Verification items for the finished model (mm, model axes). A direction names the side the tool comes from. Coordinates: 2 decimals unless noted, no trailing zeros. Order: outer loops, then holes, each group sorted by start corner. A loop starts at its lowest first (then second) coordinate and runs counter-clockwise, first axis right, second up. Notation, with made-up numbers: (63.25, 78.25) -> (104.25, 78.25) arc R29 cw to (104.25, 100.25) -> close; hole circle Ø3 at (-6, 8.25). An arc over 180 degrees is marked (long way). Answer as CSV lines item,"result".
```python
from build123d import *

# Parameters (mm, degrees)
F0_W      = 100
F0_H      = 100
F1_DEPTH  = 2
F2_R      = 7.5
F2_W      = 50.5
F2_H      = 2.1
F3_DEPTH  = 25
F4_W      = 8.5
F4_H      = 100
F4_W_2    = 3.5
F4_H_2    = 49
F5_DEPTH  = 25
F6_W      = 8.5
F6_H      = 8.5
F7_DEPTH  = 56.75
F8_W      = 2.5
F8_H      = 50
F9_DEPTH  = 5.2
F10_R     = 1
F11_W     = 1
F11_H     = 2.1
F11_W_2   = 3.33
F12_DEPTH = 4.5


# Not quite as in the source:
# - a pattern or mirror of a feature is missing from the dataset's text; its kind, count and spacing are read off the source's solid


with BuildPart() as f1:
    # F0 (on Top) → F1 (new body)
    with BuildSketch(Plane.XY):
        Rectangle(F0_W, F0_H)
    extrude(amount=F1_DEPTH)

    # F2 (on face) → F3 (cut)
    with BuildSketch(Plane.XY.offset(2)):
        with BuildLine():
            ThreePointArc((-21.1883002739, 41.0541145875), (-23.9038135596, 39.3292567737), (-23.4967439726, 36.1381063176))
            Line((-23.4967439726, 36.1381063176), (-8.2072148474, 17.7169868897))
            ThreePointArc((-8.2072148474, 17.7169868897), (-6.7654738079, 16.7609181236), (-5.0355363465, 16.7598739167))
            ThreePointArc((-5.0355363465, 16.7598739167), (0, 17.5), (5.0355363465, 16.7598739167))
            ThreePointArc((5.0355363465, 16.7598739167), (6.7654738079, 16.7609181236), (8.2072148474, 17.7169868897))
            Line((8.2072148474, 17.7169868897), (23.4967439726, 36.1381063176))
            ThreePointArc((23.4967439726, 36.1381063176), (23.9038135596, 39.3292567737), (21.1883002739, 41.0541145875))
            Line((21.1883002739, 41.0541145875), (-21.1883002739, 41.0541145875))
        make_face()
        with BuildLine():
            ThreePointArc((-15.5455239175, -8.0365842327), (-17.5, 0), (-15.5455239175, 8.0365842327))
            ThreePointArc((-15.5455239175, 8.0365842327), (-15.2278910436, 9.7371118179), (-15.9020271762, 11.3302926568))
            Line((-15.9020271762, 11.3302926568), (-31.1915563014, 29.7514120847))
            ThreePointArc((-31.1915563014, 29.7514120847), (-34.5184961718, 30.6572233604), (-36.5, 27.8354038148))
            Line((-36.5, 27.8354038148), (-36.5, -27.8354038148))
            ThreePointArc((-36.5, -27.8354038148), (-34.5184961718, -30.6572233604), (-31.1915563014, -29.7514120847))
            Line((-31.1915563014, -29.7514120847), (-15.9020271762, -11.3302926568))
            ThreePointArc((-15.9020271762, -11.3302926568), (-15.2278910436, -9.7371118179), (-15.5455239175, -8.0365842327))
        make_face()
        Circle(F2_R)
        with BuildLine():
            Line((15.9020271762, -11.3302926568), (31.1915563014, -29.7514120847))
            ThreePointArc((31.1915563014, -29.7514120847), (34.5184961718, -30.6572233604), (36.5, -27.8354038148))
            Line((36.5, -27.8354038148), (36.5, 27.8354038148))
            ThreePointArc((36.5, 27.8354038148), (34.5184961718, 30.6572233604), (31.1915563014, 29.7514120847))
            Line((31.1915563014, 29.7514120847), (15.9020271762, 11.3302926568))
            ThreePointArc((15.9020271762, 11.3302926568), (15.2278910436, 9.7371118179), (15.5455239175, 8.0365842327))
            ThreePointArc((15.5455239175, 8.0365842327), (17.5, 0), (15.5455239175, -8.0365842327))
            ThreePointArc((15.5455239175, -8.0365842327), (15.2278910436, -9.7371118179), (15.9020271762, -11.3302926568))
        make_face()
        with BuildLine():
            ThreePointArc((21.1883002739, -41.0541145875), (23.9038135596, -39.3292567737), (23.4967439726, -36.1381063176))
            Line((23.4967439726, -36.1381063176), (8.2072148474, -17.7169868897))
            ThreePointArc((8.2072148474, -17.7169868897), (6.7654738079, -16.7609181236), (5.0355363465, -16.7598739167))
            ThreePointArc((5.0355363465, -16.7598739167), (0, -17.5), (-5.0355363465, -16.7598739167))
            ThreePointArc((-5.0355363465, -16.7598739167), (-6.7654738079, -16.7609181236), (-8.2072148474, -17.7169868897))
            Line((-8.2072148474, -17.7169868897), (-23.4967439726, -36.1381063176))
            ThreePointArc((-23.4967439726, -36.1381063176), (-23.9038135596, -39.3292567737), (-21.1883002739, -41.0541145875))
            Line((-21.1883002739, -41.0541145875), (21.1883002739, -41.0541145875))
        make_face()
        with Locations((0, 48.95)):
            Rectangle(F2_W, F2_H)
        with Locations((0, -48.95)):
            Rectangle(F2_W, F2_H)
    extrude(amount=-F3_DEPTH, mode=Mode.SUBTRACT)

    # F4 (on face) → F5 (cut)
    with BuildSketch(Plane(origin=(0, 0, 0), x_dir=(1, 0, 0), z_dir=(0, 0, -1))):
        with Locations((-45.75, 0)):
            Rectangle(F4_W, F4_H)
        Polygon((50, 50), (41.5, 50), (41.5, 24.5), (46.5, 24.5), (50, 24.5), align=None)
        with Locations((48.25, 0)):
            Rectangle(F4_W_2, F4_H_2)
        Polygon((41.5, -24.5), (41.5, -50), (50, -50), (50, -24.5), (46.5, -24.5), align=None)
    extrude(amount=-F5_DEPTH, mode=Mode.SUBTRACT)

    # F6 (on Front) → F7 (join, symmetric)
    with BuildSketch(Plane.XZ):
        with Locations((-45.75, 2.25)):
            Rectangle(F6_W, F6_H)
    extrude(amount=F7_DEPTH, both=True)

    # F8 (on face) → F9 (cut)
    with BuildSketch(Plane.XY.offset(6.5)):
        with Locations((-47.03, 0)):
            Rectangle(F8_W, F8_H)
    extrude(amount=-F9_DEPTH, mode=Mode.SUBTRACT)

    # F10
    f10_edges = [f1.edges().sort_by_distance(p)[0] for p in [
        (-41.5, 0, -2),
        (-41.5, 0, 6.5),
        (-50, 0, -2),
        (-50, 0, 6.5),
    ]]
    fillet(f10_edges, radius=F10_R)

    # F11 (on face) → F12 (cut, through all)
    with BuildSketch(Plane.XY.offset(6.5)):
        with Locations((-42, 48.95)):
            Rectangle(F11_W, F11_H)
        with Locations((-44.165, 48.95)):
            Rectangle(F11_W_2, F11_H)
    f12 = extrude(amount=-F12_DEPTH, mode=Mode.SUBTRACT)

    # F12_copies: F12 across plane
    add(f12.mirror(Plane(origin=(0, 0, 0), x_dir=(0, 0, -1), z_dir=(0, -1, 0))), mode=Mode.SUBTRACT)


solid = f1.part
```
Item 1: Depth check by flat-ended pin: pin 1 Ø6 at (x, y) = (-26, 37) entering from -Z; pin 2 Ø1 at (x, z) = (-23.5, 0.5) entering from +Y; pin 3 Ø2.5 at (y, z) = (48.5, 4) entering from +X. Enter the tip coordinate at first touch or a pass-through.
Answer list:
pin 1,"z = 0"
pin 2,"y = 47.9"
pin 3,"x = -41.5"
Item 2: Section check B-B, the plane y = 0. Record the boundary of the cut face in (x, z), plus the area to 3 significant figures.
Answer list:
outline,"(-50, -1) arc R1 ccw to (-49, -2) -> (-42.5, -2) arc R1 ccw to (-41.5, -1) -> (-41.5, 0) -> (-36.5, 0) -> (-36.5, 2) -> (-41.5, 2) -> (-41.5, 5.5) arc R1 ccw to (-42.5, 6.5) -> (-45.78, 6.5) -> (-45.78, 1.3) -> (-48.28, 1.3) -> (-48.28, 6.5) -> (-49, 6.5) arc R1 ccw to (-50, 5.5) -> close; (-17.5, 0) -> (-7.5, 0) -> (-7.5, 2) -> (-17.5, 2) -> close; (7.5, 0) -> (17.5, 0) -> (17.5, 2) -> (7.5, 2) -> close; (36.5, 0) -> (46.5, 0) -> (46.5, 2) -> (36.5, 2) -> close"
area,"128 mm2"
Item 3: Section check C-C, the plane x = 27.5. Record the boundary of the cut face in (y, z).
Answer list:
outline,"(-50, 0) -> (-25.3, 0) -> (-25.3, 2) -> (-50, 2) -> close; (25.3, 0) -> (50, 0) -> (50, 2) -> (25.3, 2) -> close"
Item 4: Release check for a two-part mould opening along X. For faces 5 (the flat face through (-44, -47.9, 4)), 6 (the flat face through (-50, -1, 2)), 7 (the cylindrical face through (-7.493, 0.33, 1.014)), 8 (the flat face through (-41.5, -1, 4)) record: +X half, -X half, draft (parallel to the pull), parting line (faces both ways), or undercut.
Answer list:
face 5,"draft"
face 6,"-X half"
face 7,"undercut"
face 8,"+X half"
Item 5: Section check A-A, the plane x = 0. Record the boundary of the cut face in (y, z), plus the area to 3 significant figures.
Answer list:
outline,"(-47.9, 0) -> (-41.05, 0) -> (-41.05, 2) -> (-47.9, 2) -> close; (-17.5, 0) -> (-7.5, 0) -> (-7.5, 2) -> (-17.5, 2) -> close; (7.5, 0) -> (17.5, 0) -> (17.5, 2) -> (7.5, 2) -> close; (41.05, 0) -> (47.9, 0) -> (47.9, 2) -> (41.05, 2) -> close"
area,"67.4 mm2"
Item 6: Thickness scan on line 1 (X direction, y = 10, z = 5); line 2 (Y direction, x = -21, z = 0.5); line 3 (Z direction, x = -12.5, y = -45). Record the ranges inside material, lowest first.
Answer list:
line 1,"-50 to -48.28, -45.78 to -41.5"
line 2,"-47.9 to -41.05, -33.13 to -17.47, 17.47 to 33.13, 41.05 to 47.9"
line 3,"0 to 2"
Item 7: Tool access check on faces 1 (the flat face through (-47, -25, 4)), 2 (the flat face through (-45, -1, 6.5)), 3 (the flat face through (-23.44, 20.41, 1.01)), 4 (the flat face through (12, 1, 0)). Record the directions out of +Z, -Z, +X, -X, +Y, -Y that give a thin tool (end or side, any length) a straight path to the whole face; none if there is none.
Answer list:
face 1,"+Z"
face 2,"+Z, +X, -X, +Y, -Y"
face 3,"+Z, -Z"
face 4,"-Z, +X, +Y, -Y"
Item 8: Section check D-D, the plane y = -37.5. Record the boundary of the cut face in (x, z).
Answer list:
outline,"(-50, -1) arc R1 ccw to (-49, -2) -> (-42.5, -2) arc R1 ccw to (-41.5, -1) -> (-41.5, 0) -> (-24.14, 0) -> (-24.14, 2) -> (-41.5, 2) -> (-41.5, 5.5) arc R1 ccw to (-42.5, 6.5) -> (-49, 6.5) arc R1 ccw to (-50, 5.5) -> close; (24.14, 0) -> (41.5, 0) -> (41.5, 2) -> (24.14, 2) -> close"
